Geometry check sheet. Reference: drawing and pictorial views, mm from the part's lowest x, y, z. A direction names the side the tool comes from. Round coordinates to 2 decimals unless told otherwise and drop trailing zeros. Write each loop counter-clockwise with the first axis right and the second up, starting at its lowest first coordinate (ties: lowest second). Pieces come first, ordered by that corner, then holes. Notation, with made-up numbers: M 70.5,-38.75 L 83.5,-38.75 A10 ccw 83.5,-28.75 Z; hole C -4,3.25 d5. An arc over 180 degrees is marked long. Answer in a Markdown table with one row per item. Add a question column.
1. Material ranges on probe 1 along Y at (x, z) = (30, 22); probe 2 along Y at (x, z) = (45.5, 3), recorded low to high.
2. Sectioned sample at A-A on x = 30.48. Record the cut outline in (y, z) (3 decimals), plus the area to 3 significant figures.
3. Set-up check for the marked faces 1 and 2: record each of +Z, -Z, +X, -X, +Y, -Y from which the full face is reachable in a straight line by a thin tool's end or side.
4. Go/stop test with flat-tipped pins: pin 1 Ø2 at (x, z) = (44, 24.5) entering from -Y; pin 2 Ø4 at (y, z) = (43, 27) entering from -X; pin 3 Ø8 at (x, z) = (46, 22.5) entering from +Y. Record where each tip stops, or that it passes through.
5. Sectioned sample at C-C on z = 9. Record the cut outline in (x, y), plus the area to 3 significant figures.
6. Sectioned sample at D-D on z = 29.5. Record the cut outline in (x, y), plus the area to 3 significant figures.
7. Draft check along X on the marked faces 3, 4 and 5. Enter one of: pulls with the +X half, pulls with the -X half, needs draft (parallel to the pull), parting line crosses it, or undercut.
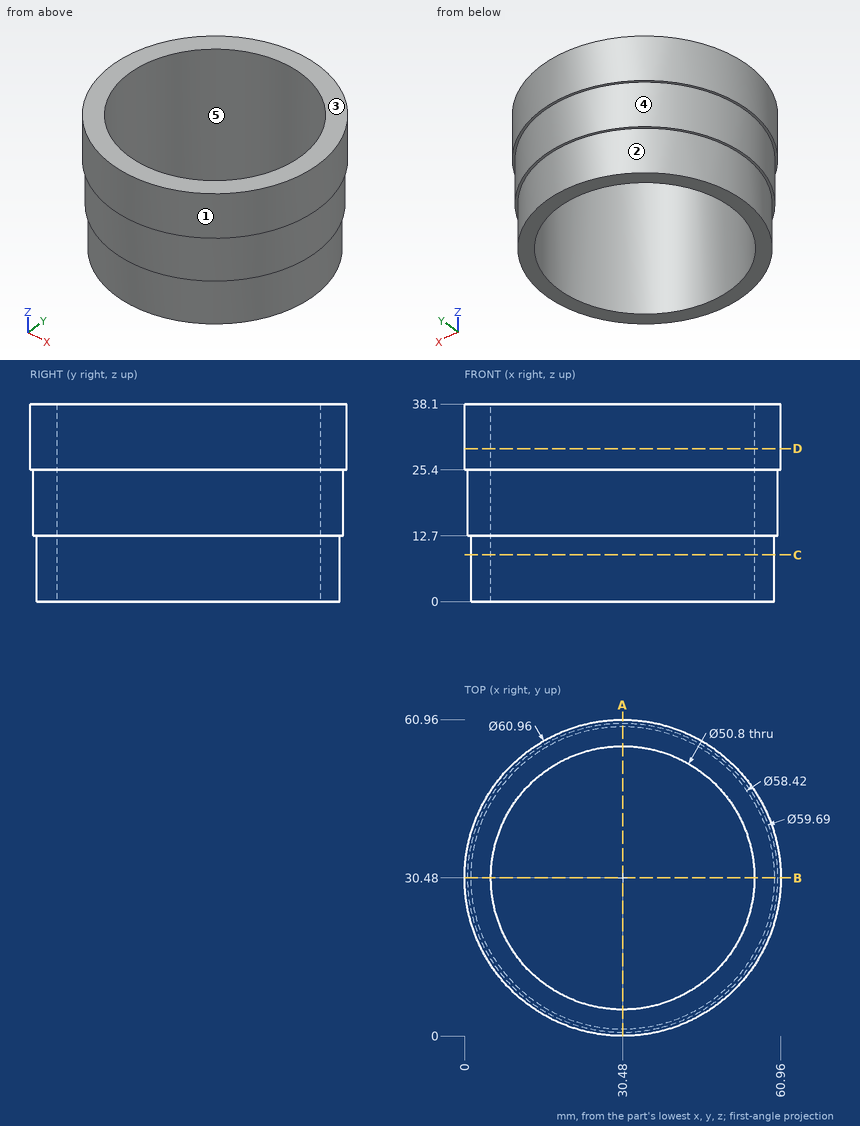
Geometry check:
| question | item | result |
|---|---|---|
| 1 | probe 1 | y = 0.64 to 5.08, 55.88 to 60.32 |
| 1 | probe 2 | y = 5.43 to 10, 50.96 to 55.53 |
| 2 | outline | M 0,25.4 L 0.635,25.4 L 0.635,12.7 L 1.27,12.7 L 1.27,0 L 5.08,0 L 5.08,38.1 L 0,38.1 Z; M 55.88,0 L 59.69,0 L 59.69,12.7 L 60.325,12.7 L 60.325,25.4 L 60.96,25.4 L 60.96,38.1 L 55.88,38.1 Z |
| 2 | area | 339 mm2 |
| 3 | face 1 | +Z, -Z |
| 3 | face 2 | -Z |
| 4 | pin 1 | stops at y = 2.95 |
| 4 | pin 2 | stops at x = 1.87 |
| 4 | pin 3 | stops at y = 58.16 |
| 5 | outline | C 30.48,30.48 d58.42; hole C 30.48,30.48 d50.8 |
| 5 | area | 654 mm2 |
| 6 | outline | C 30.48,30.48 d60.96; hole C 30.48,30.48 d50.8 |
| 6 | area | 892 mm2 |
| 7 | face 3 | needs draft |
| 7 | face 4 | parting line crosses it |
| 7 | face 5 | undercut |
